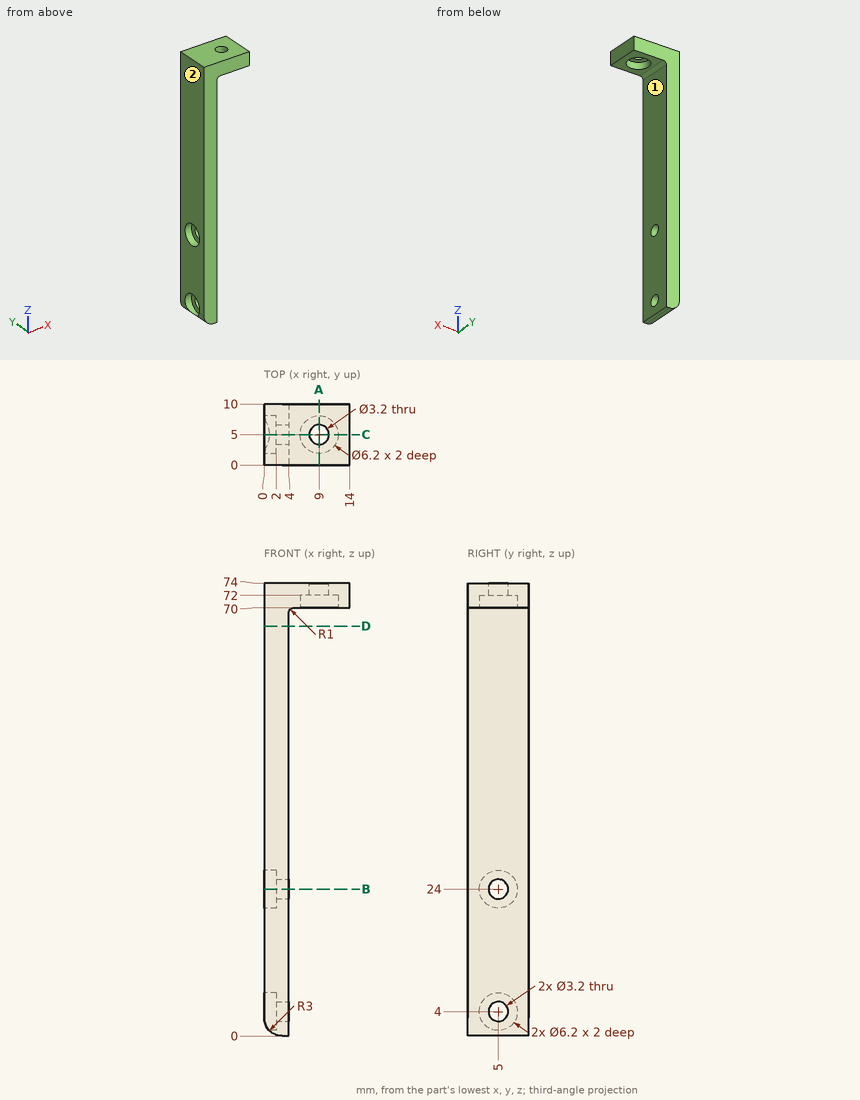
For this review, use the dimensioned drawing (mm, ordinates from the lowest corner) and the shaded views. A direction names the side the tool comes from. Round coordinates to 2 decimals unless told otherwise and drop trailing zeros. Order: outer loops, then holes, each group sorted by start corner. A loop starts at its lowest first (then second) coordinate and runs counter-clockwise, first axis right, second up. Notation, with made-up numbers: (-29.5, 86.25) -> (5.5, 86.25) arc R23 cw to (5.5, 118.25) -> close; hole circle Ø1 at (60.5, 87). An arc over 180 degrees is marked (long way). Put each result on its own line as item: value.
Q1. Add section C-C on y = 5. State how many separate pieces and enclosed holes the cut face has, plus the area to 3 significant figures.
Check result:
separate pieces: 4
enclosed holes: 0
area: 278 mm2
Q2. For probe 1 along Z at (x, y) = (3.3, 5); probe 2 along Z at (x, y) = (1.25, 4.5); probe 3 along Z at (x, y) = (0.4, 5), list the stretches that pass through material, from the lowest coordinate up. Write a range as [from, to].
Check result:
probe 1: [0, 2.4], [5.6, 22.4], [25.6, 74]
probe 2: [0.56, 0.94], [7.06, 20.94], [27.06, 74]
probe 3: [7.1, 20.9], [27.1, 74]
Q3. Insertion check: pin 1 Ø5 at (x, y) = (1.5, 5.5) entering from -Z; pin 2 Ø5 at (y, z) = (5, 4) entering from +X; pin 3 Ø3 at (y, z) = (4, 4.5) entering from -X; pin 4 Ø3 at (x, y) = (9, 5) entering from +Z. Each pin has a flat end and moves straight along its axis. Give the tip position at first contact, or say it passes through.
Check result:
pin 1: z = 0
pin 2: x = 4
pin 3: x = 2
pin 4: through
Q4. Add section D-D on z = 67. Write out the cut boundary in (x, y).
Check result:
outline: (0, 0) -> (4, 0) -> (4, 10) -> (0, 10) -> close
Q5. Machinability: for the marked faces 1 and 2, which of the approach directions +Z, -Z, +X, -X, +Y, -Y give a long, thin tool a straight path to every point of the face, cutting with its end or side? Answer none if there is none.
Check result:
face 1: -Z, +X, +Y, -Y
face 2: +Z, -Z, -X, +Y, -Y
Q6. Add section A-A on x = 9. Write out the cut boundary in (y, z).
Check result:
outline: (0, 70) -> (1.9, 70) -> (1.9, 72) -> (3.4, 72) -> (3.4, 74) -> (0, 74) -> close; (6.6, 72) -> (8.1, 72) -> (8.1, 70) -> (10, 70) -> (10, 74) -> (6.6, 74) -> close
Q7. Add section B-B on z = 24. Write out the cut boundary in (x, y).
Check result:
outline: (0, 0) -> (4, 0) -> (4, 3.4) -> (2, 3.4) -> (2, 1.9) -> (0, 1.9) -> close; (0, 8.1) -> (2, 8.1) -> (2, 6.6) -> (4, 6.6) -> (4, 10) -> (0, 10) -> close
